Check sheet for the modelled part. Datum: model origin and axes. Units: mm. A direction names the side the tool comes from. Round coordinates to 2 decimals unless told otherwise and drop trailing zeros. Order: outer loops, then holes, each group sorted by start corner. A loop starts at its lowest first (then second) coordinate and runs counter-clockwise, first axis right, second up.
Q1. Cross-section at A-A on z = 80. Record the cut outline in (x, y) (3 decimals), then the cut area to 3 significant figures.
Q2. Depth check by flat-ended pin: P1, Ø4, axis at y = 958.5, z = -102.5, coming from the -X side; P2, Ø1, axis at x = -541.5, y = 961.5, coming from the -Z side; P3, Ø1, axis at x = -527, z = 127.5, coming from the -Y side; P4, Ø10, axis at x = -603, z = -130, coming from the -Y side. Enter the tip coordinate at first touch or a pass-through.
Q3. Set-up check for faces 1 (the cylindrical face through (-606.44, 959.57, 2.31)), 2 (the flat face through (-502, 962.43, 2)): record each of +Z, -Z, +X, -X, +Y, -Y from which the full face is reachable in a straight line by a thin tool's end or side.
Q4. Scan lines: probe 1 along Y at (x, z) = (-573, -113.5); probe 2 along X at (y, z) = (949, 124); probe 3 along Y at (x, z) = (-595, -28). Record each from-to range of solid material in increasing order.
Q5. Cross-section at B-B on x = -517. Record the cut outline in (y, z), then the cut area to 3 significant figures.
from build123d import *

# Parameters (mm, degrees)
EXTRUDE_THIN1_DEPTH = 165.1


with BuildPart() as part:
    # Sketch1 → Extrude-Thin1 (new body, symmetric)
    with BuildSketch(Plane.XY):
        with BuildLine():
            Line((-418.175, 963.93), (-584.2, 963.93))
            ThreePointArc((-584.2, 963.93), (-606.742034443, 959.446110563), (-625.852248486, 946.677073774))
            Line((-625.852248486, 946.677073774), (-624.791588314, 945.616413602))
            ThreePointArc((-624.791588314, 945.616413602), (-606.168009294, 958.060291265), (-584.2, 962.43))
            Line((-584.2, 962.43), (-418.175, 962.43))
            Line((-418.175, 962.43), (-418.175, 963.93))
        make_face()
    extrude(amount=EXTRUDE_THIN1_DEPTH, both=True)


solid = part.part
Results found:
1. outline: (-625.852, 946.677) - (-624.792, 945.616) arc R57.405 cw to (-584.2, 962.43) - (-418.175, 962.43) - (-418.175, 963.93) - (-584.2, 963.93) arc R58.905 ccw to start
1. area: 318 mm2
2. P1: stops at x = -612.84
2. P2: passes through
2. P3: stops at y = 962.43
2. P4: stops at y = 957.26
3. face 1: +Z, -Z, -X, +Y
3. face 2: +Z, -Z, +X, -Y
4. probe 1: y = 962.43 to 963.93
4. probe 2: x = -623.39 to -621.1
4. probe 3: y = 961.4 to 962.93
5. outline: (962.43, -165.1) - (963.93, -165.1) - (963.93, 165.1) - (962.43, 165.1) - close
5. area: 495 mm2
